Build history of the part. All positions in model axes, mm. A direction names the side the tool comes from. Round coordinates to 2 decimals unless told otherwise and drop trailing zeros. Write each loop counter-clockwise with the first axis right and the second up, starting at its lowest first coordinate (ties: lowest second). Pieces come first, ordered by that corner, then holes. Notation, with made-up numbers: (59.25, 11.5) -> (94.25, 11.5) arc R12 cw to (94.25, 21.5) -> close; hole circle Ø11 at (9.25, -9). An arc over 180 degrees is marked (long way). Answer in a Markdown table with one row per item.
```python
from build123d import *

# Parameters (mm, degrees)
SKETCH1_R           = 5
SKETCH1_R_2         = 4
BOSS_EXTRUDE1_DEPTH = 15.6
SKETCH2_R           = 11.1
SKETCH2_R_2         = 5
SKETCH2_R_3         = 1.778
BOSS_EXTRUDE2_DEPTH = 3.683
SKETCH3_OUTSIDE_W   = 31.212
SKETCH3_OUTSIDE_H   = 31.212
CUT_EXTRUDE1_DEPTH  = 14.849999944


with BuildPart() as part:
    # Sketch1 → Boss-Extrude1 (new body)
    with BuildSketch(Plane(origin=(0, 0, 0), x_dir=(1, 0, 0), z_dir=(0, 1, 0))):
        Circle(SKETCH1_R)
        Circle(SKETCH1_R_2, mode=Mode.SUBTRACT)
    extrude(amount=BOSS_EXTRUDE1_DEPTH)

    # Sketch2 → Boss-Extrude2 (add)
    with BuildSketch(Plane(origin=(0, 1.750000056, 0), x_dir=(-1, 0, 0), z_dir=(0, -1, 0))):
        Circle(SKETCH2_R)
        Circle(SKETCH2_R_2, mode=Mode.SUBTRACT)
        with Locations((0, 7.874)):
            Circle(SKETCH2_R_3, mode=Mode.SUBTRACT)
        with Locations((7.874, 0)):
            Circle(SKETCH2_R_3, mode=Mode.SUBTRACT)
        with Locations((0, -7.874)):
            Circle(SKETCH2_R_3, mode=Mode.SUBTRACT)
        with Locations((-7.874, 0)):
            Circle(SKETCH2_R_3, mode=Mode.SUBTRACT)
    extrude(amount=-BOSS_EXTRUDE2_DEPTH)

    # Sketch3 outside → Cut-Extrude1 (cut, through all)
    with BuildSketch(Plane.XZ.offset(-1.750000056)):
        Rectangle(SKETCH3_OUTSIDE_W, SKETCH3_OUTSIDE_H)
        Polygon((0.010892417, -12.202255907), (16.316615828, 4.103467504), (4.103467504, 16.316615828), (-15.606056949, -3.392908624), (-3.392908624, -15.606056949), align=None, mode=Mode.SUBTRACT)
    extrude(amount=-CUT_EXTRUDE1_DEPTH, mode=Mode.SUBTRACT)


solid = part.part
```
Q1. Saw through at B-B on x = 0. Write the cut outline in (y, z), plus the area to 3 significant figures.
A:
| item | result |
|---|---|
| outline | (0, -5) -> (1.75, -5) -> (1.75, -6.1) -> (5.43, -6.1) -> (5.43, -5) -> (15.6, -5) -> (15.6, -4) -> (0, -4) -> close; (0, 4) -> (15.6, 4) -> (15.6, 5) -> (5.43, 5) -> (5.43, 6.1) -> (1.75, 6.1) -> (1.75, 5) -> (0, 5) -> close; (1.75, -11.1) -> (5.43, -11.1) -> (5.43, -9.65) -> (1.75, -9.65) -> close; (1.75, 9.65) -> (5.43, 9.65) -> (5.43, 11.1) -> (1.75, 11.1) -> close |
| area | 49.9 mm² |
Q2. Saw through at C-C on x = 6.75. Write the cut outline in (y, z).
A:
| item | result |
|---|---|
| outline | (1.75, -5.46) -> (5.43, -5.46) -> (5.43, -1.38) -> (1.75, -1.38) -> close; (1.75, 1.38) -> (5.43, 1.38) -> (5.43, 8.81) -> (1.75, 8.81) -> close |
Q3. Saw through at D-D on z = 6.5. Write the cut outline in (x, y).
A:
| item | result |
|---|---|
| outline | (-5.71, 1.75) -> (-1.13, 1.75) -> (-1.13, 5.43) -> (-5.71, 5.43) -> close; (1.13, 1.75) -> (9, 1.75) -> (9, 5.43) -> (1.13, 5.43) -> close |
Q4. Wall check: line 1 (X direction, y = 4.45, z = 0); line 2 (Z direction, x = 0, y = 12). Give the ranges that are in metal, low to high. Write a range as [from, to].
A:
| item | result |
|---|---|
| line 1 | [-11.1, -9.65], [-6.1, -4], [4, 6.1], [9.65, 11.1] |
| line 2 | [-5, -4], [4, 5] |
Q5. Two-plate mould, pull along X, no slides. Class faces 4 (the cylindrical face through (0.39, 3.57, 9.61)), 5 (the flat face through (-5, 5.433, 2)), 6 (the flat face through (-6.038, 3.566, 6.176)), 7 (the flat face through (6.038, 3.566, -6.176)): released by +X, released by -X, zero draft, split by the parting line, or undercut.
A:
| item | result |
|---|---|
| face 4 | undercut |
| face 5 | zero draft |
| face 6 | released by -X |
| face 7 | released by +X |
Q6. Drop flat-ended pins along their axis: P1, Ø6.5, axis at x = 2.5, z = -5, coming from the +Y side; P2, Ø3, axis at x = 7.874, z = 0, coming from the -Y side; P3, Ø5.5, axis at x = 0, z = 7.874, coming from the +Y side; P4, Ø5, axis at x = 7, y = 2, coming from the +Z side. Give the stop position or say it passes through.
A:
| item | result |
|---|---|
| P1 | y = 15.6 |
| P2 | through |
| P3 | y = 5.43 |
| P4 | z = 10.15 |
Q7. Saw through at A-A on z = 0. Write the cut outline in (x, y).
A:
| item | result |
|---|---|
| outline | (-11.1, 1.75) -> (-9.65, 1.75) -> (-9.65, 5.43) -> (-11.1, 5.43) -> close; (-6.1, 1.75) -> (-5, 1.75) -> (-5, 0) -> (-4, 0) -> (-4, 15.6) -> (-5, 15.6) -> (-5, 5.43) -> (-6.1, 5.43) -> close; (4, 0) -> (5, 0) -> (5, 1.75) -> (6.1, 1.75) -> (6.1, 5.43) -> (5, 5.43) -> (5, 15.6) -> (4, 15.6) -> close; (9.65, 1.75) -> (11.1, 1.75) -> (11.1, 5.43) -> (9.65, 5.43) -> close |
Q8. Which spindle directions (+Z, -Z, +X, -X, +Y, -Y) get a long thin tool onto all of the face, cutting with end or side? Do faces 1 (the cylindrical face through (-1.08, 10.45, 4.88)), 2 (the cylindrical face through (6.178, 3.566, -0.534)), 3 (the cylindrical face through (-1.08, 0.86, 4.88)). Say none if no direction does.
A:
| item | result |
|---|---|
| face 1 | +Y |
| face 2 | +Y, -Y |
| face 3 | -Y |
